```python
from build123d import *

# Parameters (mm, degrees)
SKETCH1_W           = 19.05
SKETCH1_H           = 2.54
SKETCH1_H_2         = 3.175
BOSS_EXTRUDE1_DEPTH = 1.524


with BuildPart() as part:
    # Sketch1 → Boss-Extrude1 (new body)
    with BuildSketch(Plane(origin=(0, 0, 0), x_dir=(1, 0, 0), z_dir=(0, 1, 0))):
        with Locations((15.24, -7.3025)):
            Rectangle(SKETCH1_W, SKETCH1_H)
        Polygon((5.715, -6.0325), (5.715, 5.3975), (5.715, 8.5725), (-5.715, 8.5725), (-5.715, -8.5725), (5.715, -8.5725), align=None)
        with Locations((15.24, 6.985)):
            Rectangle(SKETCH1_W, SKETCH1_H_2)
    extrude(amount=BOSS_EXTRUDE1_DEPTH)


solid = part.part
```
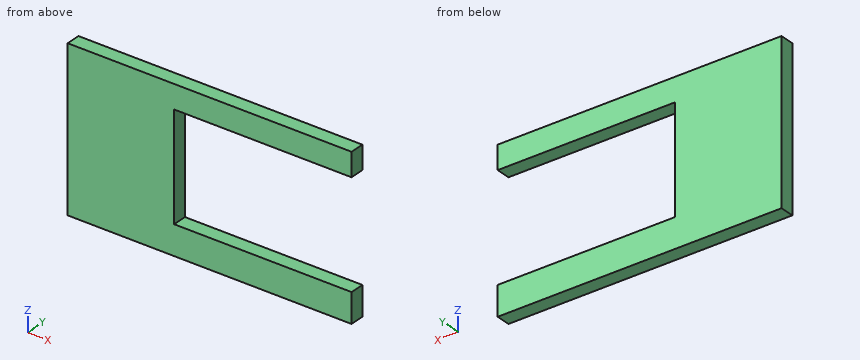
Could you check a few things on this model? Use its own coordinates, in mm. Give positions to 0.01 mm unless a question says otherwise; leave off trailing zeros. Loops run counter-clockwise (first coordinate to the right, second up) from the corner with the lowest first, then second, coordinate; pieces in that order, holes last. Notation, with made-up numbers: (-8, -11.5) - (19, -11.5) arc R37 cw to (19, 24.5) - close; hole circle Ø5 at (17, 63). An arc over 180 degrees is marked (long way). Answer in a Markdown table with one row per item. Add a question column.
Q1. Please list where these lines run through material, in increasing order: L1, parallel to Z at x = 20, y = 1.4; L2, parallel to X at y = 1.05, z = 1 (3 decimals). Write a range as from..to.
Q2. If we section it at A-A (x = 8): List the corners of the cut face in (y, z) for me.
Q3. For pin 1 (0.8 mm diameter, centred on y = 0.5, z = 0.5, fed in from +X) (3 decimals), with a flat end and sliding along its axis, tell me the tip position at first contact or that it passes through.
Q4. If we section it at C-C (z = -2.25): List the corners of the cut face in (x, y) for me (3 decimals), plus the area to 3 significant figures.
Q5. If we section it at B-B (y = 0.3): List the corners of the cut face in (x, z) for me (1 decimal).
The answers:
| question | item | result |
|---|---|---|
| 1 | L1 | z = -8.57..-5.4, 6.03..8.57 |
| 1 | L2 | x = -5.715..5.715 |
| 2 | outline | (0, -8.57) - (1.52, -8.57) - (1.52, -5.4) - (0, -5.4) - close; (0, 6.03) - (1.52, 6.03) - (1.52, 8.57) - (0, 8.57) - close |
| 3 | pin 1 | stops at x = 5.715 |
| 4 | outline | (-5.715, 0) - (5.715, 0) - (5.715, 1.524) - (-5.715, 1.524) - close |
| 4 | area | 17.4 mm^2 |
| 5 | outline | (-5.7, -8.6) - (24.8, -8.6) - (24.8, -5.4) - (5.7, -5.4) - (5.7, 6) - (24.8, 6) - (24.8, 8.6) - (-5.7, 8.6) - close |
